Read the model definition and answer for the solid it produces. Units are mm, in the model's axes. A direction names the side the tool comes from. Coordinates: 2 decimals unless noted, no trailing zeros. Loops run counter-clockwise (first coordinate to the right, second up) from the corner with the lowest first, then second, coordinate; pieces in that order, holes last. Notation, with made-up numbers: M 88.5,-36 L 95.5,-36 A24 ccw 95.5,-2 Z; hole C 29,-7 d4. An arc over 180 degrees is marked long. One line per item, written item: value. Start each with the question number.
1. Determine the mould class of faces 5 (the face through (-24.233, 7.368, -25.439)), 6 (the face through (26, 4, -21.4)) for opening direction X: +X half, -X half, draft (parallel to the pull), parting line (faces both ways), or undercut.
2. Flat-ended cylindrical pins translate along their axes: pin 1 (2 mm diameter, centred on y = -1.5, z = 7.5, fed in from -X); pin 2 (4.5 mm diameter, centred on x = -25.5, z = -25, fed in from +Y); pin 3 (10 mm diameter, centred on x = 18, z = -3, fed in from +Y); pin 4 (1.5 mm diameter, centred on y = 2.5, z = 1.5, fed in from -X). Find the tip coordinate at first contact, or state that the pin passes through.
3. The part is cut by section A-A (y = 2.6). Write down the section's boundary in (x, z).
4. For faces 1 (the face through (26, 4, 3)), 2 (the face through (-26, 4, 3)), 3 (the face through (27, 0.5, -25)), 4 (the face through (24.216, 7.368, -25.411)), determine the directions among +Z, -Z, +X, -X, +Y, -Y from which every point of the face is accessible in a straight line to the end or side of a thin tool.
5. The part is cut by section B-B (x = -10). Write down the section's boundary in (y, z), then the cut area to 3 significant figures.
6. The part is cut by section C-C (x = 26). Write down the section's boundary in (y, z).
7. Consider probe 1 along Z at (x, y) = (-26, 3); probe 2 along Y at (x, z) = (-2.5, -16); probe 3 along Z at (x, y) = (-21, 3). Determine where each line is inside the solid, lowest interval first.
```python
from build123d import *

# Parameters (mm, degrees)
ESBO_O1_W                 = 58
ESBO_O1_H                 = 6
RESSALTO_EXTRUS_O1_DEPTH  = 8.6
ESBO_O2_W                 = 47.9
ESBO_O2_H                 = 6
RESSALTO_EXTRUS_O2_DEPTH  = 3.4
CORTE_EXTRUS_O2_DEPTH     = 7
ESBO_O8_W                 = 5.05
ESBO_O8_H                 = 6
CORTE_EXTRUS_O3_DEPTH     = 0.5
ESBO_O9_W                 = 46
ESBO_O9_H                 = 2
CORTE_EXTRUS_O4_DEPTH     = 8.1
ESBO_O10_W                = 47.9
ESBO_O10_H                = 2
CORTE_EXTRUS_O5_DEPTH     = 3.9
ESBO_O11_W                = 0.95
ESBO_O11_H                = 4
CORTE_EXTRUS_O6_DEPTH     = 4.9
ESBO_O15_W                = 4
ESBO_O15_H                = 3.9
RESSALTO_EXTRUS_O4_DEPTH  = 0.17
ESBO_O16_R                = 1
CORTE_EXTRUS_O9_DEPTH     = 2.5
ESBO_O16_4_R              = 1
CORTE_EXTRUS_O10_DEPTH    = 13
RESSALTO_EXTRUS_O5_DEPTH  = 14.2
ESBO_O18_W                = 2
ESBO_O18_H                = 8.1
CORTE_EXTRUS_O11_DEPTH    = 0.17
ESBO_O19_W                = 2
ESBO_O19_H                = 8.1
CORTE_EXTRUS_O12_DEPTH    = 0.17
ESBO_O20_W                = 4
ESBO_O20_H                = 3.9
RESSALTO_EXTRUS_O6_DEPTH  = 0.17
ESBO_O23_W                = 6
ESBO_O23_H                = 8.1
RESSALTO_EXTRUS_O9_DEPTH  = 0.17
ESBO_O24_W                = 6
ESBO_O24_H                = 8.1
RESSALTO_EXTRUS_O10_DEPTH = 0.17


with BuildPart() as part:
    # Esboço1 → Ressalto-extrusão1 (new body)
    with BuildSketch(Plane(origin=(0, 0, 0), x_dir=(1, 0, 0), z_dir=(0, 1, 0))):
        Rectangle(ESBO_O1_W, ESBO_O1_H)
    extrude(amount=RESSALTO_EXTRUS_O1_DEPTH)

    # Esboço2 → Ressalto-extrusão2 (add)
    with BuildSketch(Plane.XZ):
        Rectangle(ESBO_O2_W, ESBO_O2_H)
    extrude(amount=RESSALTO_EXTRUS_O2_DEPTH)

    # Esboço4 → Corte-extrusão2 (cut, through all)
    with BuildSketch(Plane.XY.offset(3)):
        with BuildLine():
            Line((-17, 4.6), (17, 4.6))
            ThreePointArc((17, 4.6), (19, 2.6), (17, 0.6))
            Line((17, 0.6), (-17, 0.6))
            ThreePointArc((-17, 0.6), (-19, 2.6), (-17, 4.6))
        make_face()
    extrude(amount=-CORTE_EXTRUS_O2_DEPTH, mode=Mode.SUBTRACT)


with BuildPart() as body_2:
    # Espelhar1: mirrored copy
    add(part.part.mirror(Plane(origin=(-29, 8.6, 3), x_dir=(1, 0, 0), z_dir=(0, 0, -1))))

    # Esboço8 → Corte-extrusão3 (cut)
    with BuildSketch(Plane.XZ):
        with Locations((-26.475, 6)):
            Rectangle(ESBO_O8_W, ESBO_O8_H)
        with Locations((26.475, 6)):
            Rectangle(ESBO_O8_W, ESBO_O8_H)
    extrude(amount=-CORTE_EXTRUS_O3_DEPTH, mode=Mode.SUBTRACT)

    # Esboço9 → Corte-extrusão4 (cut)
    with BuildSketch(Plane(origin=(0, 8.6, 0), x_dir=(1, 0, 0), z_dir=(0, 1, 0))):
        with Locations((0, -4)):
            Rectangle(ESBO_O9_W, ESBO_O9_H)
    extrude(amount=-CORTE_EXTRUS_O4_DEPTH, mode=Mode.SUBTRACT)

    # Esboço10 → Corte-extrusão5 (cut)
    with BuildSketch(Plane.XZ.offset(3.4)):
        with Locations((0, 4)):
            Rectangle(ESBO_O10_W, ESBO_O10_H)
    extrude(amount=-CORTE_EXTRUS_O5_DEPTH, mode=Mode.SUBTRACT)

    # Esboço11 → Corte-extrusão6 (cut, through all)
    with BuildSketch(Plane.XZ.offset(-0.5)):
        with Locations((23.475, 7)):
            Rectangle(ESBO_O11_W, ESBO_O11_H)
        with Locations((-23.475, 7)):
            Rectangle(ESBO_O11_W, ESBO_O11_H)
    extrude(amount=CORTE_EXTRUS_O6_DEPTH, mode=Mode.SUBTRACT)

    # Esboço15 → Ressalto-extrusão4 (add)
    with BuildSketch(Plane.ZY.offset(23)):
        with Locations((7, -1.45)):
            Rectangle(ESBO_O15_W, ESBO_O15_H)
    extrude(amount=RESSALTO_EXTRUS_O4_DEPTH)

    # Esboço16 → Corte-extrusão9 (cut)
    with BuildSketch(Plane(origin=(0, 8.6, 0), x_dir=(1, 0, 0), z_dir=(0, 1, 0))):
        with Locations((26, -6)):
            Circle(ESBO_O16_R)
        Polygon((27.183568052, -3.95), (24.816431948, -3.95), (23.632863896, -6), (24.816431948, -8.05), (27.183568052, -8.05), (28.367136104, -6), align=None)
        with Locations((26, -6)):
            Circle(ESBO_O16_R, mode=Mode.SUBTRACT)
        Polygon((-24.816431948, -3.95), (-27.183568052, -3.95), (-28.367136104, -6), (-27.183568052, -8.05), (-24.816431948, -8.05), (-23.632863896, -6), align=None)
        with Locations((-26, -6)):
            Circle(ESBO_O16_R, mode=Mode.SUBTRACT)
        with Locations((-26, -6)):
            Circle(ESBO_O16_R)
    extrude(amount=-CORTE_EXTRUS_O9_DEPTH, mode=Mode.SUBTRACT)

    # Esboço16<4> → Corte-extrusão10 (cut, through all)
    with BuildSketch(Plane(origin=(0, 8.6, 0), x_dir=(1, 0, 0), z_dir=(0, 1, 0))):
        with Locations((26, -6)):
            Circle(ESBO_O16_4_R)
        with Locations((-26, -6)):
            Circle(ESBO_O16_4_R)
    extrude(amount=-CORTE_EXTRUS_O10_DEPTH, mode=Mode.SUBTRACT)

    # Esboço17 → Ressalto-extrusão5 (add)
    with BuildSketch(Plane(origin=(0, 0, 5), x_dir=(-1, 0, 0), z_dir=(0, 0, -1))):
        with BuildLine():
            Line((17, 5.6), (-17, 5.6))
            ThreePointArc((-17, 5.6), (-20, 2.6), (-17, -0.4))
            Line((-17, -0.4), (17, -0.4))
            ThreePointArc((17, -0.4), (20, 2.6), (17, 5.6))
        make_face()
        with BuildLine():
            Line((-17, 0.6), (17, 0.6))
            ThreePointArc((17, 0.6), (19, 2.6), (17, 4.6))
            Line((17, 4.6), (-17, 4.6))
            ThreePointArc((-17, 4.6), (-19, 2.6), (-17, 0.6))
        make_face(mode=Mode.SUBTRACT)
    extrude(amount=RESSALTO_EXTRUS_O5_DEPTH)

    # Esboço18 → Corte-extrusão11 (cut)
    with BuildSketch(Plane(origin=(-23, 0, 0), x_dir=(0, 0, -1), z_dir=(1, 0, 0))):
        with Locations((-4, 4.55)):
            Rectangle(ESBO_O18_W, ESBO_O18_H)
    extrude(amount=-CORTE_EXTRUS_O11_DEPTH, mode=Mode.SUBTRACT)

    # Esboço19 → Corte-extrusão12 (cut)
    with BuildSketch(Plane.ZY.offset(-23)):
        with Locations((4, 4.55)):
            Rectangle(ESBO_O19_W, ESBO_O19_H)
    extrude(amount=-CORTE_EXTRUS_O12_DEPTH, mode=Mode.SUBTRACT)

    # Esboço20 → Ressalto-extrusão6 (add)
    with BuildSketch(Plane(origin=(23, 0, 0), x_dir=(0, 0, -1), z_dir=(1, 0, 0))):
        with Locations((-7, -1.45)):
            Rectangle(ESBO_O20_W, ESBO_O20_H)
    extrude(amount=RESSALTO_EXTRUS_O6_DEPTH)

    # Esboço23 → Ressalto-extrusão9 (add)
    with BuildSketch(Plane.ZY.offset(29)):
        with Locations((6, 4.55)):
            Rectangle(ESBO_O23_W, ESBO_O23_H)
    extrude(amount=RESSALTO_EXTRUS_O9_DEPTH)

    # Esboço24 → Ressalto-extrusão10 (add)
    with BuildSketch(Plane(origin=(29, 0, 0), x_dir=(0, 0, -1), z_dir=(1, 0, 0))):
        with Locations((-6, 4.55)):
            Rectangle(ESBO_O24_W, ESBO_O24_H)
    extrude(amount=RESSALTO_EXTRUS_O10_DEPTH)

    # Espelhar2: body 2 across plane


with BuildPart() as body_2_1:
    add(body_2.part)
    add(body_2.part.mirror(Plane(origin=(-17, 2.6, -9.2), x_dir=(1, 0, 0), z_dir=(0, 0, -1))))


solid = body_2_1.part
```
Answer block:
1. face 5: undercut
1. face 6: draft
2. pin 1: stops at x = -23.17
2. pin 2: stops at y = 8.6
2. pin 3: stops at y = 5.6
2. pin 4: stops at x = -20
3. outline: M -29.17,-27.4 L -19,-27.4 L -19,9 L -29.17,9 L -29.17,3 L -23.17,3 L -23.17,5 L -20,5 L -20,-23.4 L -23.17,-23.4 L -23.17,-21.4 L -29.17,-21.4 Z; M 19,-27.4 L 29.17,-27.4 L 29.17,-21.4 L 23.17,-21.4 L 23.17,-23.4 L 20,-23.4 L 20,5 L 23.17,5 L 23.17,3 L 29.17,3 L 29.17,9 L 19,9 Z; hole C -26,-24.4 d2; hole C -26,6 d2; hole C 26,-24.4 d2; hole C 26,6 d2
4. face 1: +X, +Y, -Y
4. face 2: -X, +Y, -Y
4. face 3: +Z, -Z, +X, -Y
4. face 4: +Y
5. outline: M -3.4,-27.4 L 0.6,-27.4 L 0.6,9 L -3.4,9 L -3.4,5 L -0.4,5 L -0.4,-23.4 L -3.4,-23.4 Z; M 4.6,-27.4 L 8.6,-27.4 L 8.6,-23.4 L 5.6,-23.4 L 5.6,5 L 8.6,5 L 8.6,9 L 4.6,9 Z
5. area: 121 mm2
6. outline: M 0.5,-27.4 L 8.6,-27.4 L 8.6,-26.45 L 6.1,-26.45 L 6.1,-25.4 L 0.5,-25.4 Z; M 0.5,-23.4 L 6.1,-23.4 L 6.1,-22.35 L 8.6,-22.35 L 8.6,-21.4 L 0.5,-21.4 Z; M 0.5,3 L 8.6,3 L 8.6,3.95 L 6.1,3.95 L 6.1,5 L 0.5,5 Z; M 0.5,7 L 6.1,7 L 6.1,8.05 L 8.6,8.05 L 8.6,9 L 0.5,9 Z
7. probe 1: z = -27.4 to -25.4, -23.4 to -21.4, 3 to 5, 7 to 9
7. probe 2: y = -0.4 to 0.6, 4.6 to 5.6
7. probe 3: z = -27.4 to -23.4, 5 to 9
